from build123d import *

# Parameters (mm, degrees)
BOSS_EXTRUDE1_DEPTH          = 2
BOSS_EXTRUDE2_DEPTH          = 2
SKETCH4_R                    = 2.5
CUT_EXTRUDE2_DEPTH           = 2
CSK_FOR_M5_SFHCS1_AT_2_COUNT = 2
CSK_FOR_M5_SFHCS1_AT_2_PITCH = 44.45
CSK_FOR_M5_SFHCS1_AT_3_COUNT = 2
CSK_FOR_M5_SFHCS1_AT_3_PITCH = 42.64624896
CSK_FOR_M5_SFHCS1_AT_4_COUNT = 2
CSK_FOR_M5_SFHCS1_AT_4_PITCH = 20


with BuildPart() as part:
    # Sketch2 → Boss-Extrude1 (new body)
    with BuildSketch(Plane.XY):
        Polygon((-54.61917065, -24.589230235), (30.72482935, -24.589230235), (13.852659447, -75.725684813), (-71.491340553, -75.725684813), align=None)
    extrude(amount=BOSS_EXTRUDE1_DEPTH)

    # Sketch3 → Boss-Extrude2 (add)
    with BuildSketch(Plane.XY.offset(2)):
        Polygon((-72.764711867, -79.585039875), (11.90144755, -81.639450446), (13.852659447, -75.725684813), (-71.491340553, -75.725684813), align=None)
    extrude(amount=-BOSS_EXTRUDE2_DEPTH)

    # Sketch4 → Cut-Extrude2 (cut)
    with BuildSketch(Plane.XY.offset(2)):
        with Locations((-32.900665919, -39.829230235)):
            Circle(SKETCH4_R)
        with Locations((11.549334081, -39.829230235)):
            Circle(SKETCH4_R)
        with Locations((5.282742972, -58.822119322)):
            Circle(SKETCH4_R)
        with Locations((-39.167257028, -58.822119322)):
            Circle(SKETCH4_R)
    extrude(amount=-CUT_EXTRUDE2_DEPTH, mode=Mode.SUBTRACT)

    # Sketch6 → CSK for M5 SFHCS1 (revolve, cut)
    with BuildSketch(Plane(origin=(-32.900665919, -39.829230235, 2), x_dir=(0, -1, 0), z_dir=(1, 0, 0))):
        Polygon((0, 0), (0, 2), (2.75, 2), (2.75, 2.85), (5.6, 0), align=None)
    csk_for_m5_sfhcs1 = revolve(axis=Axis((-32.900665919, -39.829230235, 8.35), (0, 0, -1)), mode=Mode.SUBTRACT)

    # CSK for M5 SFHCS1 at 2: CSK for M5 SFHCS1 ×2
    with Locations(*[(i * CSK_FOR_M5_SFHCS1_AT_2_PITCH, 0, 0) for i in range(1, CSK_FOR_M5_SFHCS1_AT_2_COUNT)]):
        add(csk_for_m5_sfhcs1, mode=Mode.SUBTRACT)

    # CSK for M5 SFHCS1 at 3: CSK for M5 SFHCS1 ×2
    with Locations(*[Vector(0.8953521076667903, -0.44535896004979675, 0) * (i * CSK_FOR_M5_SFHCS1_AT_3_PITCH) for i in range(1, CSK_FOR_M5_SFHCS1_AT_3_COUNT)]):
        add(csk_for_m5_sfhcs1, mode=Mode.SUBTRACT)

    # CSK for M5 SFHCS1 at 4: CSK for M5 SFHCS1 ×2
    with Locations(*[Vector(-0.31332955547970925, -0.9496444543421964, 0) * (i * CSK_FOR_M5_SFHCS1_AT_4_PITCH) for i in range(1, CSK_FOR_M5_SFHCS1_AT_4_COUNT)]):
        add(csk_for_m5_sfhcs1, mode=Mode.SUBTRACT)


solid = part.part
Geometry: final body of the model. Coordinates: model frame, mm. Coordinates: 2 decimals unless noted, no trailing zeros. Order: outer loops, then holes, each group sorted by start corner. A loop starts at its lowest first (then second) coordinate and runs counter-clockwise, first axis right, second up. Notation, with made-up numbers: M 3.25,85.25 L 37.25,85.25 A18 ccw 37.25,105.25 Z; hole C -4.5,80.5 d9. An arc over 180 degrees is marked long. One line per question, with ' | ' between items. Start each with the question number.
Item 1: Ray query, probe 1 along Y at (x, z) = (1, 1.15); probe 2 along Y at (x, z) = (-34, 0.5); probe 3 along Z at (x, y) = (1.5, -56). Return the intervals inside material, ascending. Write a range as [from, to].
Item 2: Cut plane B-B, the plane y = -40. Count the separate pieces of the cut face and the enclosed holes in it, then the cut area to 3 significant figures.
Item 3: Cut plane C-C, the plane y = -68. Return the cut outline in (x, z).
Item 4: Cut plane D-D, the plane x = -65.5. Return the cut outline in (y, z).
Item 5: Cut plane A-A, the plane z = 0.85. Return the cut outline in (x, y), then the cut area to 3 significant figures.
A:
1) probe 1: y = [-81.37, -60.88], [-56.77, -24.59] | probe 2: y = [-80.53, -43.78], [-35.88, -24.59] | probe 3: z = [0, 1.12]
2) separate pieces: 3 | enclosed holes: 0 | area: 134 mm2
3) outline: M -68.94,0 L 16.4,0 L 16.4,2 L -68.94,2 Z
4) outline: M -79.76,0 L -57.57,0 L -57.57,2 L -79.76,2 Z
5) outline: M -72.76,-79.59 L 11.9,-81.64 L 30.72,-24.59 L -54.62,-24.59 Z; hole C -39.17,-58.82 d8.9; hole C -32.9,-39.83 d8.9; hole C 5.28,-58.82 d8.9; hole C 11.55,-39.83 d8.9 | area: 4,530 mm2
